Could you check a few things on this model? Use its own coordinates, in mm. A direction names the side the tool comes from. Give positions to 0.01 mm unless a question says otherwise; leave off trailing zeros. Write each loop counter-clockwise with the first axis right and the second up, starting at its lowest first coordinate (ties: lowest second). Pieces come first, ordered by that corner, then holes. Notation, with made-up numbers: (-31.5, 38.5) - (-6.5, 38.5) arc R23 cw to (-6.5, 56.5) - close; hole circle Ø6 at (86.25, 26.25). An arc over 180 degrees is marked (long way). Answer in a Markdown table with one row per item.
from build123d import *

# Parameters (mm, degrees)
F0_W     = 175.017152
F0_H     = 175.017152
F0_R     = 1.7272
F0_R_2   = 9.525
F1_DEPTH = 5.08


with BuildPart() as f1:
    # F0 (on Top) → F1 (new body)
    with BuildSketch(Plane.XY):
        Rectangle(F0_W, F0_H)
        with Locations((-81.158576, -82.746076)):
            Circle(F0_R, mode=Mode.SUBTRACT)
        with Locations((-81.158576, -63.696076)):
            Circle(F0_R, mode=Mode.SUBTRACT)
        with Locations((-10.664054, -10.664054)):
            Circle(F0_R, mode=Mode.SUBTRACT)
        with Locations((81.158576, -82.746076)):
            Circle(F0_R, mode=Mode.SUBTRACT)
        with Locations((81.158576, -63.696076)):
            Circle(F0_R, mode=Mode.SUBTRACT)
        with Locations((10.664054, -10.664054)):
            Circle(F0_R, mode=Mode.SUBTRACT)
        with Locations((-10.664054, 10.664054)):
            Circle(F0_R, mode=Mode.SUBTRACT)
        with Locations((-81.158576, 63.696076)):
            Circle(F0_R, mode=Mode.SUBTRACT)
        with Locations((-81.158576, 82.746076)):
            Circle(F0_R, mode=Mode.SUBTRACT)
        with Locations((-24.892, 53.050918)):
            Circle(F0_R, mode=Mode.SUBTRACT)
        with Locations((-24.892, 62.829918)):
            Circle(F0_R, mode=Mode.SUBTRACT)
        Circle(F0_R_2, mode=Mode.SUBTRACT)
        with Locations((10.664054, 10.664054)):
            Circle(F0_R, mode=Mode.SUBTRACT)
        with BuildLine():
            Line((-20.32, 58.956418), (-20.32, 67.719418))
            Line((-20.32, 67.719418), (20.32, 67.719418))
            Line((20.32, 67.719418), (20.32, 58.956418))
            Line((20.32, 58.956418), (23.749, 58.956418))
            ThreePointArc((23.749, 58.956418), (24.765, 57.940418), (23.749, 56.924418))
            Line((23.749, 56.924418), (20.32, 56.924418))
            Line((20.32, 56.924418), (20.32, 48.161418))
            Line((20.32, 48.161418), (-20.32, 48.161418))
            Line((-20.32, 48.161418), (-20.32, 56.924418))
            Line((-20.32, 56.924418), (-23.749, 56.924418))
            ThreePointArc((-23.749, 56.924418), (-24.765, 57.940418), (-23.749, 58.956418))
            Line((-23.749, 58.956418), (-20.32, 58.956418))
        make_face(mode=Mode.SUBTRACT)
        with Locations((24.892, 53.050918)):
            Circle(F0_R, mode=Mode.SUBTRACT)
        with Locations((24.892, 62.829918)):
            Circle(F0_R, mode=Mode.SUBTRACT)
        with Locations((81.158576, 63.696076)):
            Circle(F0_R, mode=Mode.SUBTRACT)
        with Locations((81.158576, 82.746076)):
            Circle(F0_R, mode=Mode.SUBTRACT)
    extrude(amount=F1_DEPTH)


solid = f1.part
1) On a 3-axis mill with a long thin cutter (end or side, diameter ignored), from which of +Z, -Z, +X, -X, +Y, -Y can I reach the whole of each face in a straight line? I mean faces 5 (the face through (-87.509, -1, 3)), 6 (the face through (0, 67.719, 3)). Say none if no direction works.
Check values:
| item | result |
|---|---|
| face 5 | +Z, -Z, -X, +Y, -Y |
| face 6 | +Z, -Z |
2) Imagine slicing it at B-B (y = 0). List the corners of the cut face in (x, z) for me (3 decimals), then the cut area to 3 significant figures.
Check values:
| item | result |
|---|---|
| outline | (-87.509, 0) - (-9.525, 0) - (-9.525, 5.08) - (-87.509, 5.08) - close; (9.525, 0) - (87.509, 0) - (87.509, 5.08) - (9.525, 5.08) - close |
| area | 792 mm2 |
3) We'd pull the mould along Y, two halves only. Please class faces 1 (the face through (87.509, -1, 3)), 2 (the face through (-7.559, -5.796, 2.504)), 3 (the face through (-1, -87.509, 3)), 4 (the face through (-1, 87.509, 3)): +Y half, -Y half, draft (parallel to the pull), parting line (faces both ways), or undercut.
Check values:
| item | result |
|---|---|
| face 1 | draft |
| face 2 | undercut |
| face 3 | -Y half |
| face 4 | +Y half |
4) Imagine slicing it at A-A (x = -17). List the corners of the cut face in (y, z) for me.
Check values:
| item | result |
|---|---|
| outline | (-87.51, 0) - (48.16, 0) - (48.16, 5.08) - (-87.51, 5.08) - close; (67.72, 0) - (87.51, 0) - (87.51, 5.08) - (67.72, 5.08) - close |
5) Imagine slicing it at C-C (z = 3.75). State how many separate pieces and enclosed holes the cut face has, then the cut area to 3 significant figures.
Check values:
| item | result |
|---|---|
| separate pieces | 1 |
| enclosed holes | 18 |
| area | 29,400 mm2 |
6) Will this pin go through, and if not, where does the flat tip stop? P1, Ø4, axis at x = 24.89, y = 53.05, coming from the +Z side.
Check values:
| item | result |
|---|---|
| P1 | stops at z = 5.08 |
7) If I drill on line 1 (Y direction, x = 0, z = 2.3) (3 decimals); line 2 (X direction, y = 11.5, z = 1.1); line 3 (Y direction, x = -7, z = 4), over which ranges is the centre line in solid material (lowest first)?
Check values:
| item | result |
|---|---|
| line 1 | y = -87.509 to -9.525, 9.525 to 48.161, 67.719 to 87.509 |
| line 2 | x = -87.51 to -12.18, -9.15 to 9.15, 12.18 to 87.51 |
| line 3 | y = -87.51 to -6.46, 6.46 to 48.16, 67.72 to 87.51 |
